from build123d import *

# Parameters (mm, degrees)
F0_R          = 25.4
F1_DEPTH      = 50.8
F2_R          = 25.4
F3_R          = 25.39999
F4_W          = 7.62
F4_H          = 10.16
F4_W_2        = 7.6200046011
F5_DEPTH      = 50.8
F6_W          = 21.59
F6_H          = 14.5421422695
F7_DEPTH      = 61.976
F7_DEPTH_BACK = 25.4
F8_R          = 7.62
F9_R          = 7.62
F10_W         = 2.54
F10_H         = 79.756
F11_DEPTH     = 25.4
F12_W         = 38.1
F12_H         = 20.32
F13_DEPTH     = 76.2
F15_DEPTH     = 25.4


# Not quite as in the source:
# - a fillet or chamfer is up to 0.001 mm smaller than in the source, because OpenCascade refuses the exact size


with BuildPart() as f1:
    # F0 (on Front) → F1 (new body)
    with BuildSketch(Plane.XZ):
        Circle(F0_R)
    extrude(amount=F1_DEPTH)

    # F2
    f2_edges = [f1.edges().sort_by_distance(p)[0] for p in [
        (-25.4, -50.8, 0),
    ]]
    fillet(f2_edges, radius=F2_R)

    # F3 (radius 25.4 in the source; OpenCascade refuses exactly that, so slightly less here)
    f3_edges = [f1.edges().sort_by_distance(p)[0] for p in [
        (-25.4, 0, 0),
    ]]
    fillet(f3_edges, radius=F3_R)

    # F4 (on Top) → F5 (join)
    with BuildSketch(Plane.XY):
        with Locations((3.81, -23.7836401282)):
            Rectangle(F4_W, F4_H)
        with Locations((-3.8100023006, -23.7836401282)):
            Rectangle(F4_W_2, F4_H)
    extrude(amount=F5_DEPTH)

    # F6 (on face) → F7 (join, two sides)
    with BuildSketch(Plane.XY.offset(50.8)) as f7_sk:
        Polygon((7.62, -33.2457823977), (7.62, -18.7036401282), (29.21, -18.7036401282), (29.21, -12.9257823977), (-29.21, -12.9257823977), (-29.21, -18.7036401282), (-29.21, -33.2457823977), align=None)
        with Locations((18.415, -25.9747112629)):
            Rectangle(F6_W, F6_H)
    extrude(amount=F7_DEPTH)
    extrude(f7_sk.sketch, amount=-F7_DEPTH_BACK)

    # F8
    f8_edges = [f1.edges().sort_by_distance(p)[0] for p in [
        (29.21, -23.085782, 25.4),
    ]]
    fillet(f8_edges, radius=F8_R)

    # F9
    f9_edges = [f1.edges().sort_by_distance(p)[0] for p in [
        (-29.21, -23.085782, 25.4),
    ]]
    fillet(f9_edges, radius=F9_R)

    # F10 (on face) → F11 (cut)
    with BuildSketch(Plane.XZ.offset(33.2457823977)):
        with Locations((20.32, 72.898)):
            Rectangle(F10_W, F10_H)
        with Locations((-20.32, 72.898)):
            Rectangle(F10_W, F10_H)
    extrude(amount=-F11_DEPTH, mode=Mode.SUBTRACT)

    # F12 (on face) → F13 (join)
    with BuildSketch(Plane.XY.offset(112.776)):
        with Locations((0, -23.0857823977)):
            Rectangle(F12_W, F12_H)
    extrude(amount=F13_DEPTH)

    # F14 (on face) → F15 (cut)
    with BuildSketch(Plane(origin=(0, -12.9257823977, 0), x_dir=(-1, 0, 0), z_dir=(0, 1, 0))):
        Polygon((-2.54, 188.976), (0, 112.776), (0, 188.976), align=None)
        Polygon((0, 188.976), (0, 112.776), (2.54, 188.976), align=None)
    extrude(amount=-F15_DEPTH, mode=Mode.SUBTRACT)


solid = f1.part
Could you check a few things on this model? Use its own coordinates, in mm. A direction names the side the tool comes from. Give positions to 0.01 mm unless a question says otherwise; leave off trailing zeros. Loops run counter-clockwise (first coordinate to the right, second up) from the corner with the lowest first, then second, coordinate; pieces in that order, holes last. Notation, with made-up numbers: (15.25, 1.25) -> (69.25, 1.25) arc R15 cw to (69.25, 15.25) -> close; hole circle Ø9 at (84.25, 19). An arc over 180 degrees is marked (long way). Return JSON: item names as keys, results as strings.
Item 1: If we section it at C-C on y = -37.5: List the corners of the cut face in (x, z) for me.
Geometry results:
{"outline": "circle Ø44.67 at (0, 0)"}
Item 2: I need wall thicknesses on L1, parallel to X at y = -23, z = 45; L2, parallel to Y at x = -11, z = 131.5; L3, parallel to X at y = -15.5, z = 141.5. Which ranges of each line are inside material? Lowest first, please. Write a range as from..to.
Geometry results:
{"L1": "x = -29.21..-21.59, -19.05..19.05, 21.59..29.21", "L2": "y = -33.25..-12.93", "L3": "x = -19.05..-0.96, 0.96..19.05"}
Item 3: If we section it at A-A on z = 57: List the corners of the cut face in (x, y) for me, plus the area to 3 significant figures.
Geometry results:
{"outline": "(-29.21, -33.25) -> (-21.59, -33.25) -> (-21.59, -12.93) -> (-29.21, -12.93) -> close; (-19.05, -33.25) -> (19.05, -33.25) -> (19.05, -12.93) -> (-19.05, -12.93) -> close; (21.59, -33.25) -> (29.21, -33.25) -> (29.21, -12.93) -> (21.59, -12.93) -> close", "area": "1,080 mm²"}
Item 4: We'd pull the mould along Z, two halves only. Please class faces 4 (the flat face through (-25, -23, 112.776)), 5 (the flat face through (-29.21, -23, 73)), 6 (the flat face through (0, -18, 25.4)): +Z half, -Z half, draft (parallel to the pull), parting line (faces both ways), or undercut.
Geometry results:
{"face 4": "+Z half", "face 5": "draft", "face 6": "undercut"}
Item 5: I'm going to push flat-ended pins straight in: pin 1 (2.5 mm diameter, centred on x = -27, y = -21.5, fed in from +Z); pin 2 (4 mm diameter, centred on x = -13.5, y = -31.5, fed in from -Z); pin 3 (10 mm diameter, centred on x = 18, z = 24, fed in from +Y). Where does each tip first touch, or does it pass through?
Geometry results:
{"pin 1": "stops at z = 112.78", "pin 2": "stops at z = -21.93", "pin 3": "stops at y = -12.93"}
Item 6: If we section it at B-B on y = -45.5: List the corners of the cut face in (x, z) for me, plus the area to 3 significant figures.
Geometry results:
{"outline": "circle Ø31.06 at (0, 0)", "area": "758 mm²"}
Item 7: Which directions (+Z, -Z, +X, -X, +Y, -Y) give clear straight access to the entire face, cutting with the end or side of a thin tool? Please do faces 1 (the flat face through (25, -23, 112.776)), 2 (the flat face through (0, -12.926, 88)), 3 (the flat face through (19.05, -23, 110)).
Geometry results:
{"face 1": "+Z, +X, +Y, -Y", "face 2": "+Z, +X, -X, +Y", "face 3": "+Z, +Y, -Y"}
